Source: CAD feature listing. Evaluate the final solid. Frame: model axes, mm. Face numbers are marked on the shaded views. A direction names the side the tool comes from. Coordinates: 2 decimals unless noted, no trailing zeros. Loops run counter-clockwise (first coordinate to the right, second up) from the corner with the lowest first, then second, coordinate; pieces in that order, holes last. Notation, with made-up numbers: M 30.5,-4.5 L 86.5,-4.5 A21 cw 86.5,0.5 Z; hole C -17,-17.5 d10. An arc over 180 degrees is marked long. One line per question, with ' | ' between items. Start each with the question number.
1. Pin query (flat end, axial travel): P1, Ø4, axis at x = 100, y = 0, coming from the +Z side; P2, Ø2, axis at y = 2, z = 2.5, coming from the +X side; P3, Ø6, axis at x = 0, y = 5, coming from the -Z side; P4, Ø1, axis at x = 58, y = -3.5, coming from the -Z side. Return the tip coordinate at first contact, or that it passes through.
2. Section query B-B, the plane x = 0. Output: boundary loops of the cut face in (y, z), and give its area (3 significant figures).
3. Access query for the marked faces 1 and 2. Directions: +Z, -Z, +X, -X, +Y, -Y. A direction counts if a zero-diameter tool reaches every point of the face in a straight line with its end or side. Return the directions, or none.
4. Section query D-D, the plane x = 89.5. Output: boundary loops of the cut face in (y, z).
5. Ray query, probe 1 along Y at (x, z) = (0, 2.55); probe 2 along Y at (x, z) = (0, 0.5); probe 3 along Y at (x, z) = (75, 0.75). Return the intervals inside material, ascending.
6. Section query C-C, the plane z = 2. Output: boundary loops of the cut face in (x, y).
7. Section query A-A, the plane y = 0. Output: boundary loops of the cut face in (x, z).
Autodesk Inventor part; units mm, degrees
ref_plane "YZ Plane" through (0, 0, 0) normal (1, 0, 0) x (0, 1, 0)
ref_plane "XZ Plane" through (0, 0, 0) normal (0, 1, 0) x (-1, 0, 0)
ref_plane "XY Plane" through (0, 0, 0) normal (0, 0, 1) x (1, 0, 0)
sketch "スケッチ1" plane through (0, 0, 0) normal (0, 0, 1) x (1, 0, 0)
  circle A0 centre (0, 5) radius 1.55
  circle A1 centre (0, -5) radius 1.55
  line L0 (0, 5) -> (0, -5) construction
  line L1 (0, 0) -> (100, 0) construction
  circle A2 centre (100, 0) radius 1.55
  line L2 (-5, 10) -> (-5, -10)
  line L3 (-5, -10) -> (5, -10)
  line L4 (5, -10) -> (100.2521, -5.9947)
  line L5 (-5, 10) -> (5, 10)
  line L6 (5, 10) -> (100.2521, 5.9947)
  arc A3 (100.2521, -5.9947) -> (100.2521, 5.9947) centre (100, 0) ccw
  circle A4 centre (0, 5) radius 3 construction
  circle A5 centre (0, 5) radius 5 construction
  line L7 (5, 10) -> (5, -10) construction
  point P0 (-5, 0)
  dimension "d0" = 10
  dimension "d1" = 3.1
  dimension "d2" = 3.1
  dimension "d3" = 100
  dimension "d4" = 6
  dimension "d5" = 6
  dimension "d6" = 2
extrude "押し出し1" add sketch "スケッチ1" along normal blind 5
sketch "スケッチ2" plane through (0, 0, 0) normal (0, 0, -1) x (-1, 0, 0)
  circle A0 centre (-100, 0) radius 1.55
  arc A1 (-100.2521, 5.9947) -> (-100.2521, -5.9947) centre (-100, 0) ccw
  circle A2 centre (-100, 0) radius 4.05
  point P0 (0, 0)
  dimension "d9" = 8.1
extrude "押し出し2" cut sketch "スケッチ2" against normal blind 3
sketch "スケッチ3" plane through (0, 0, 0) normal (0, 0, -1) x (-1, 0, 0)
  circle A0 centre (0, -5) radius 1.55
  circle A1 centre (0, 5) radius 1.55
  line L0 (0, -1.8246) -> (2.75, -3.4123)
  line L1 (2.75, -3.4123) -> (2.75, -6.5877)
  line L2 (2.75, -6.5877) -> (0, -8.1754)
  line L3 (0, -8.1754) -> (-2.75, -6.5877)
  line L4 (-2.75, -6.5877) -> (-2.75, -3.4123)
  line L5 (-2.75, -3.4123) -> (0, -1.8246)
  line L6 (-2.75, 6.5877) -> (0, 8.1754)
  line L7 (0, 8.1754) -> (2.75, 6.5877)
  line L8 (2.75, 6.5877) -> (2.75, 3.4123)
  line L9 (2.75, 3.4123) -> (0, 1.8246)
  line L10 (0, 1.8246) -> (-2.75, 3.4123)
  line L11 (-2.75, 3.4123) -> (-2.75, 6.5877)
  line L12 (0, -8.2332) -> (2.8, -6.6166)
  line L13 (2.8, -6.6166) -> (2.8, -3.3834)
  line L14 (2.8, -3.3834) -> (0, -1.7668)
  line L15 (0, -1.7668) -> (-2.8, -3.3834)
  line L16 (-2.8, -3.3834) -> (-2.8, -6.6166)
  line L17 (-2.8, -6.6166) -> (0, -8.2332)
  line L18 (-2.8, 3.3834) -> (0, 1.7668)
  line L19 (0, 1.7668) -> (2.8, 3.3834)
  line L20 (2.8, 3.3834) -> (2.8, 6.6166)
  line L21 (2.8, 6.6166) -> (0, 8.2332)
  line L22 (0, 8.2332) -> (-2.8, 6.6166)
  line L23 (-2.8, 6.6166) -> (-2.8, 3.3834)
  circle A2 centre (0, -7.1832) radius 1.05
  circle A3 centre (1.8907, -6.0916) radius 1.05
  circle A4 centre (1.8907, -3.9084) radius 1.05
  circle A5 centre (0, -2.8168) radius 1.05
  circle A6 centre (-1.8907, -3.9084) radius 1.05
  circle A7 centre (-1.8907, -6.0916) radius 1.05
  circle A8 centre (0, 2.8168) radius 1.05
  circle A9 centre (1.8907, 3.9084) radius 1.05
  circle A10 centre (1.8907, 6.0916) radius 1.05
  circle A11 centre (0, 7.1832) radius 1.05
  circle A12 centre (-1.8907, 6.0916) radius 1.05
  circle A13 centre (-1.8907, 3.9084) radius 1.05
  circle A14 centre (0, 5) radius 3.2332
  circle A15 centre (0, -5) radius 3.2332
  point P0 (0, 0)
  point P1 (2.8, -6.6166)
  point P2 (2.8, -3.3834)
  point P3 (0, -1.7668)
  point P4 (-2.8, -3.3834)
  point P5 (-2.8, -6.6166)
  point P6 (2.8, 3.3834)
  point P7 (2.8, 6.6166)
  point P8 (0, 8.2332)
  point P9 (-2.8, 6.6166)
  point P10 (-2.8, 3.3834)
  dimension "d16" = 2.1
  dimension "d15" = 5.5
  dimension "d17" = 0.05
  dimension "d20" = 360
  dimension "d24" = 360
extrude "押し出し3" cut sketch "スケッチ3" against normal blind 1
sketch "スケッチ4" plane through (0, 0, 0) normal (0, 0, -1) x (-1, 0, 0)
  circle A0 centre (-100, 0) radius 4.05
  line L0 (-100.2521, 5.9947) -> (-5, 10)
  arc A1 (-100.2521, 5.9947) -> (-100.2521, -5.9947) centre (-100, 0) ccw
  line L1 (-5, -10) -> (-100.2521, -5.9947)
  line L2 (-7.8, -6.8796) -> (-94.9345, -3.2157)
  line L3 (-5, -10) -> (-100.2521, -5.9947)
  arc A2 (-94.9345, -3.2157) -> (-94.9345, 3.2157) centre (-100, 0) ccw
  line L4 (-94.9345, 3.2157) -> (-7.8, 6.8796)
  line L5 (-7.8, 6.8796) -> (-7.8, -6.8796)
  point P0 (-2.8, 4.4334)
  point P1 (0, 0)
  dimension "d26" = 3
  dimension "d27" = 3
  dimension "d28" = 5
extrude "押し出し4" cut sketch "スケッチ4" against normal blind 4 contours L2 A2 L4 L5
fillet "フィレット1" radius 2 4 edges at (7.8, 6.8796, 2) (7.8, -6.8796, 2) (94.9345, 3.2157, 2) (94.9345, -3.2157, 2)
equation "\"d27\" = d26"
properties part number "胴体_サブフレーム_1_12" material "アセタール樹脂、黒"
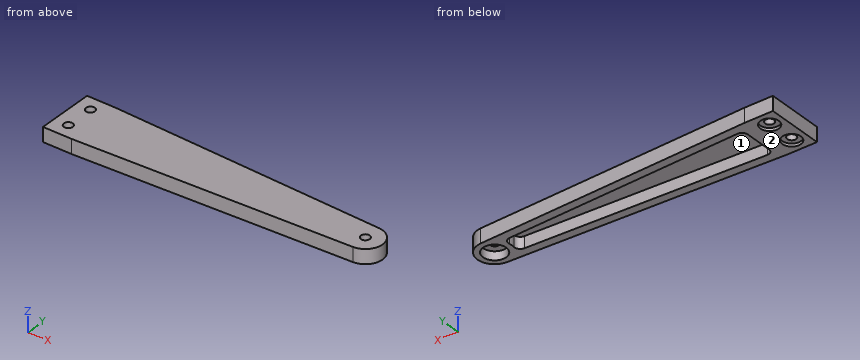
Taken from the geometry:
1) P1: z = 5 | P2: x = 105.92 | P3: z = 1 | P4: z = 4
2) outline: M -10,0 L -8.23,0 L -8.23,1 L -6.55,1 L -6.55,5 L -10,5 Z; M -3.45,1 L -1.77,1 L -1.77,0 L 1.77,0 L 1.77,1 L 3.45,1 L 3.45,5 L -3.45,5 Z; M 6.55,1 L 8.23,1 L 8.23,0 L 10,0 L 10,5 L 6.55,5 Z | area: 62.3 mm^2
3) face 1: -Z | face 2: -Z, +X, -X, +Y, -Y
4) outline: M -6.45,0 L -3.44,0 L -3.44,4 L 3.44,4 L 3.44,0 L 6.45,0 L 6.45,5 L -6.45,5 Z
5) probe 1: -10 to -6.55, -3.45 to 3.45, 6.55 to 10 | probe 2: -10 to -8.23, -1.77 to 1.77, 8.23 to 10 | probe 3: -7.06 to -4.05, 4.05 to 7.06
6) outline: M -5,-10 L 5,-10 L 100.25,-5.99 A6 ccw 100.25,5.99 L 5,10 L -5,10 Z; hole C 0,-5 d3.1; hole C 0,5 d3.1; hole M 7.8,-4.79 A2 ccw 9.88,-6.79 L 92.2,-3.33 A2 ccw 94.08,-1 A6 cw 94.08,1 A2 ccw 92.2,3.33 L 9.88,6.79 A2 ccw 7.8,4.79 Z; hole C 100,0 d8.1
7) outline: M -5,0 L 7.8,0 L 7.8,4 L 94,4 L 94,0 L 95.95,0 L 95.95,3 L 98.45,3 L 98.45,5 L -5,5 Z; M 101.55,3 L 104.05,3 L 104.05,0 L 106,0 L 106,5 L 101.55,5 Z
